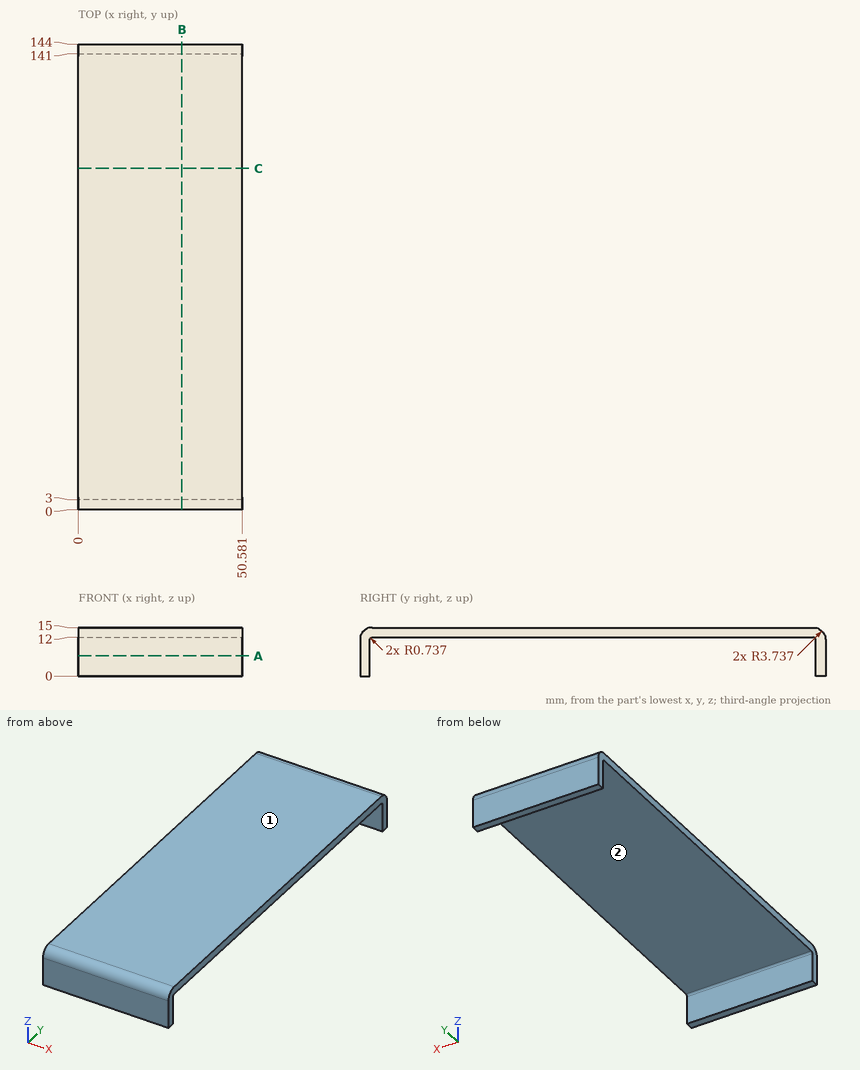
The drawing under review shows one solid part. Ordinate dimensions are in mm from its lowest x, y, z. A direction names the side the tool comes from. Round coordinates to 2 decimals unless told otherwise and drop trailing zeros. Write each loop counter-clockwise with the first axis right and the second up, starting at its lowest first coordinate (ties: lowest second). Pieces come first, ordered by that corner, then holes. Notation, with made-up numbers: (57, 24.25) -> (115, 24.25) arc R22 cw to (115, 34.25) -> close; hole circle Ø11 at (-26.75, -17). An arc over 180 degrees is marked (long way). One line per question, with ' | ' between items. Start each with the question number.
(1) Add section B-B, the plane x = 32. Write out the cut boundary in (y, z).
(2) Tool access review of the marked faces 1 and 2: name each direction out of +Z, -Z, +X, -X, +Y, -Y from which nothing blocks a thin tool from reaching the whole face with its end or side.
(3) Add section A-A, the plane z = 6.25. Write out the cut boundary in (x, y).
(4) For line 1 along Y through (x, z) = (39, 9.5); line 2 along Z through (x, y) = (15.5, 52); line 3 along Y through (x, z) = (3.5, 12.25), list the stretches that pass through material, from the lowest coordinate up. Write a range as from..to.
(5) Insertion check: P1, Ø1, axis at x = 17, y = 24.5, coming from the -Z side. The pin has a flat end and moves straight along its axis. Give the tip position at first contact, or say it passes through.
(6) Add section C-C, the plane y = 105.5. Write out the cut boundary in (x, z), plus the area to 3 significant figures.
Answer list:
1) outline: (0, 0) -> (3, 0) -> (3, 11.26) arc R0.74 cw to (3.74, 12) -> (140.26, 12) arc R0.74 cw to (141, 11.26) -> (141, 0) -> (144, 0) -> (144, 11.26) arc R3.74 ccw to (140.26, 15) -> (3.74, 15) arc R3.74 ccw to (0, 11.26) -> close
2) face 1: +Z, +X, -X, +Y, -Y | face 2: -Z, +X, -X
3) outline: (0, 0) -> (50.58, 0) -> (50.58, 3) -> (0, 3) -> close; (0, 141) -> (50.58, 141) -> (50.58, 144) -> (0, 144) -> close
4) line 1: 0..3, 141..144 | line 2: 12..15 | line 3: 0.13..143.87
5) P1: z = 12
6) outline: (0, 12) -> (50.58, 12) -> (50.58, 15) -> (0, 15) -> close | area: 152 mm²
